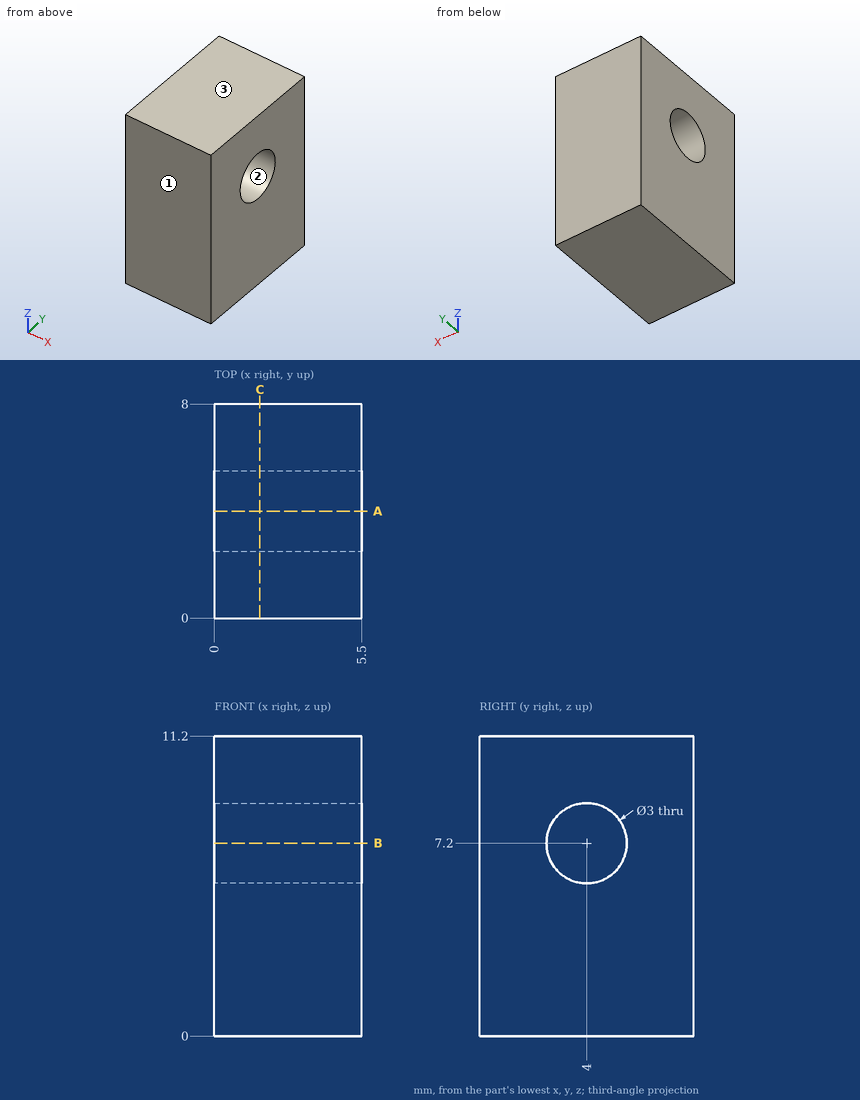
Geometry check sheet. Reference: drawing and pictorial views, mm from the part's lowest x, y, z. Coordinates: 2 decimals unless noted, no trailing zeros. Write each loop counter-clockwise with the first axis right and the second up, starting at its lowest first coordinate (ties: lowest second). Pieces come first, ordered by that corner, then holes. Notation, with made-up numbers: (-22, 17.25) - (10, 17.25) arc R19 ccw to (10, 50.25) - close; hole circle Ø11 at (81, -3.5). An arc over 180 degrees is marked (long way). One line per question, with ' | ' between items. Start each with the question number.
1. Draft check along Z on the marked faces 1, 2 and 3. Enter one of: released by +Z, released by -Z, zero draft, split by the parting line, or undercut.
2. Material ranges on line 1 along Z through (x, y) = (3.3, 4); line 2 along Y through (x, z) = (1.8, 7.2); line 3 along Z through (x, y) = (1, 5), recorded low to high.
3. Section check B-B (z = 7.2). Enter the section's corners in (x, y).
4. Section check A-A (y = 4). Enter the section's corners in (x, z), plus the area to 3 significant figures.
5. Section check C-C (x = 1.7). Enter the section's corners in (y, z).
Computed values:
1) face 1: zero draft | face 2: undercut | face 3: released by +Z
2) line 1: 0 to 5.7, 8.7 to 11.2 | line 2: 0 to 2.5, 5.5 to 8 | line 3: 0 to 6.08, 8.32 to 11.2
3) outline: (0, 0) - (5.5, 0) - (5.5, 2.5) - (0, 2.5) - close; (0, 5.5) - (5.5, 5.5) - (5.5, 8) - (0, 8) - close
4) outline: (0, 0) - (5.5, 0) - (5.5, 5.7) - (0, 5.7) - close; (0, 8.7) - (5.5, 8.7) - (5.5, 11.2) - (0, 11.2) - close | area: 45.1 mm²
5) outline: (0, 0) - (8, 0) - (8, 11.2) - (0, 11.2) - close; hole circle Ø3 at (4, 7.2)
